Could you check a few things on this model? Use its own coordinates, in mm. A direction names the side the tool comes from. Coordinates: 2 decimals unless noted, no trailing zeros. Order: outer loops, then holes, each group sorted by start corner. A loop starts at its lowest first (then second) coordinate and runs counter-clockwise, first axis right, second up.
```python
from build123d import *

# Parameters (mm, degrees)
SKETCH_1_R          = 18
EXTRUDE_1_DEPTH     = 116
CUT_EXTRUDE_START   = -38
SKETCH_2_R          = 18
SKETCH_2_R_2        = 15
CUT_EXTRUDE_1_DEPTH = 38
CUT_EXTRUDE_START_2 = -32
SKETCH_3_R          = 15
SKETCH_3_R_2        = 14
CUT_EXTRUDE_2_DEPTH = 32
SKETCH_4_R          = 18
SKETCH_4_R_2        = 15
CUT_EXTRUDE_3_DEPTH = 48
CUT_EXTRUDE_4_DEPTH = 25
FILLET_1_R          = 1
FILLET_2_R          = 1


with BuildPart() as part:
    # 草图1 → 凸台-拉伸1 (new body)
    with BuildSketch(Plane.XY):
        with Locations(Location((0, 0, 0), (0, 0, 180))):
            Circle(SKETCH_1_R)
    extrude(amount=EXTRUDE_1_DEPTH)

    # 草图2 → 切除-拉伸1 (cut)
    with BuildSketch(Plane.XY.offset(116).offset(CUT_EXTRUDE_START)):
        with Locations(Location((0, 0, 0), (0, 0, 180))):
            Circle(SKETCH_2_R)
        Circle(SKETCH_2_R_2, mode=Mode.SUBTRACT)
    extrude(amount=CUT_EXTRUDE_1_DEPTH, mode=Mode.SUBTRACT)

    # 草图3 → 切除-拉伸2 (cut)
    with BuildSketch(Plane.XY.offset(116).offset(CUT_EXTRUDE_START_2)):
        Circle(SKETCH_3_R)
        Circle(SKETCH_3_R_2, mode=Mode.SUBTRACT)
    extrude(amount=CUT_EXTRUDE_2_DEPTH, mode=Mode.SUBTRACT)

    # 草图4 → 切除-拉伸3 (cut)
    with BuildSketch(Plane(origin=(0, 0, 0), x_dir=(-1, 0, 0), z_dir=(0, 0, -1))):
        Circle(SKETCH_4_R)
        with Locations(Location((0, 0, 0), (0, 0, 180))):
            Circle(SKETCH_4_R_2, mode=Mode.SUBTRACT)
    extrude(amount=-CUT_EXTRUDE_3_DEPTH, mode=Mode.SUBTRACT)

    # 草图5 → 旋转2 (revolve)
    with BuildSketch(Plane(origin=(0, 0, 0), x_dir=(-1, 0, 0), z_dir=(0, 0, -1))):
        with BuildLine():
            Line((0, 28), (0, -28))
            Line((0, -28), (0, -38.2))
            ThreePointArc((0, -38.2), (38.2, 0), (0, 38.2))
            Line((0, 38.2), (0, 28))
        make_face()
    revolve(axis=Axis((0, 28, 0), (0, -1, 0)))

    # 草图6 → 切除-拉伸4 (cut)
    with BuildSketch(Plane(origin=(0, 0, 48), x_dir=(-1, 0, 0), z_dir=(0, 0, -1))):
        Polygon((15, 0), (15, 35.868856724), (38.265827157, 35.868856724), (38.265827157, -37.868854143), (15, -37.868854143), align=None)
        Polygon((-15, -37.868854143), (-15, 0), (-15, 35.868856724), (-38.265827157, 35.868856724), (-38.265827157, -37.868854143), align=None)
    extrude(amount=-CUT_EXTRUDE_4_DEPTH, mode=Mode.SUBTRACT)

    # 圆角1
    fillet_1_edges = [part.edges().sort_by_distance(p)[0] for p in [
        (-15, 0, 84),
        (-14, 0, 116),
        (0, 18, 48),
        (18, 0, 78),
    ]]
    fillet(fillet_1_edges, radius=FILLET_1_R - 0.0001)  # a hair under: the kernel refuses the full size

    # 圆角2
    fillet_2_edges = [part.edges().sort_by_distance(p)[0] for p in [
        (0, -18, 48),
    ]]
    fillet(fillet_2_edges, radius=FILLET_2_R)


solid = part.part
```
Item 1: I need wall thicknesses on line 1 (Y direction, x = 11.5, z = -26.5); line 2 (Z direction, x = 25, y = 2); line 3 (Y direction, x = 10, z = 108). Which ranges of each line are inside material? Lowest first, please.
Item 2: Suppose I cut it at C-C (y = 20.5). List the corners of the cut face in (x, z) for me.
Item 3: For pin 1 Ø2.5 at (x, y) = (-17, 0) entering from -Z; pin 2 Ø13.5 at (x, y) = (6, -7.5) entering from -Z; pin 3 Ø5 at (x, z) = (-3.5, 94.5) entering from +Y, each with a flat end and sliding along its axis, tell me the tip position at first contact or that it passes through.
Item 4: Suppose I cut it at B-B (z = 95.5). List the corners of the cut face in (x, y) for me.
Item 5: Thinking about a two-plate mould opening in Z: for faces 1 (the face through (-15, 0, 60)), 2 (the face through (12.932, -5.362, 99.283)), 3 (the face through (0, 0, 116)), 4 (the face through (0.1, 15.5, 48)), which applies, +Z half, -Z half, draft (parallel to the pull), parting line (faces both ways), or undercut?
Item 6: Which directions (+Z, -Z, +X, -X, +Y, -Y) give clear straight access to the entire face, cutting with the end or side of a thin tool? Please do faces 5 (the face through (13.267, -12.165, 62.804)), 6 (the face through (0.1, -15.4, 48)), 7 (the face through (15, 0, 60)), 8 (the face through (8.06, -12.65, 41.48)).
Geometry results:
1. line 1: y = -24.99 to 24.99
1. line 2: z = -28.81 to 28.81
1. line 3: y = -9.8 to 9.8
2. outline: circle Ø64.47 at (0, 0)
3. pin 1: stops at z = -34.8
3. pin 2: stops at z = -38.09
3. pin 3: stops at y = 13.96
4. outline: circle Ø28 at (0, 0)
5. face 1: undercut
5. face 2: draft
5. face 3: +Z half
5. face 4: undercut
6. face 5: +Z
6. face 6: -Y
6. face 7: +X, +Y, -Y
6. face 8: none
